CAD build for the part. Positions are in the model's coordinates, mm. A direction names the side the tool comes from. Round coordinates to 2 decimals unless told otherwise and drop trailing zeros. Loops run counter-clockwise (first coordinate to the right, second up) from the corner with the lowest first, then second, coordinate; pieces in that order, holes last. Notation, with made-up numbers: (-28.5, 79) - (-2.5, 79) arc R21 cw to (-2.5, 113) - close; hole circle Ø9 at (-7, 64). An arc over 180 degrees is marked (long way). Use one line per item in the form item = value.
from build123d import *

# Parameters (mm, degrees)
SKETCH1_W           = 53.6
SKETCH1_H           = 39.6
BOSS_EXTRUDE1_DEPTH = 2
SKETCH2_W           = 53.6
SKETCH2_H           = 39.6
SKETCH2_W_2         = 49.6
SKETCH2_H_2         = 35.6
BOSS_EXTRUDE2_DEPTH = 20
SKETCH3_W           = 70
SKETCH3_H           = 60
SKETCH3_W_2         = 49.6
SKETCH3_H_2         = 35.6
BOSS_EXTRUDE3_DEPTH = 3
CHAMFER1_SIZE       = 10
FILLET1_R           = 3


with BuildPart() as part:
    # Sketch1 → Boss-Extrude1 (new body)
    with BuildSketch(Plane(origin=(0, 0, 0), x_dir=(1, 0, 0), z_dir=(0, 1, 0))):
        Rectangle(SKETCH1_W, SKETCH1_H)
    extrude(amount=BOSS_EXTRUDE1_DEPTH)

    # Sketch2 → Boss-Extrude2 (add)
    with BuildSketch(Plane(origin=(0, 2, 0), x_dir=(1, 0, 0), z_dir=(0, 1, 0))):
        Rectangle(SKETCH2_W, SKETCH2_H)
        Rectangle(SKETCH2_W_2, SKETCH2_H_2, mode=Mode.SUBTRACT)
    extrude(amount=BOSS_EXTRUDE2_DEPTH)

    # Sketch3 → Boss-Extrude3 (add)
    with BuildSketch(Plane(origin=(0, 22, 0), x_dir=(1, 0, 0), z_dir=(0, 1, 0))):
        Rectangle(SKETCH3_W, SKETCH3_H)
        Rectangle(SKETCH3_W_2, SKETCH3_H_2, mode=Mode.SUBTRACT)
    extrude(amount=BOSS_EXTRUDE3_DEPTH)

    # Chamfer1
    chamfer1_edges = [part.edges().sort_by_distance(p)[0] for p in [
        (0, 2, -17.8),
        (0, 0, -19.8),
    ]]
    chamfer(chamfer1_edges, length=CHAMFER1_SIZE)

    # Fillet1
    fillet1_edges = [part.edges().sort_by_distance(p)[0] for p in [
        (24.8, 13.5, 17.8),
        (0, 25, 17.8),
        (-24.8, 13.5, 17.8),
        (0, 2, 17.8),
        (24.8, 18.5, -17.8),
        (-24.8, 18.5, -17.8),
        (24.8, 2, 5),
        (-24.8, 2, 5),
        (24.8, 25, 0),
        (0, 25, -17.8),
        (-24.8, 25, 0),
        (0, 25, 30),
        (0, 25, -30),
        (35, 25, 0),
        (-35, 25, 0),
        (0, 12, -17.8),
        (24.8, 7, -12.8),
        (-24.8, 7, -12.8),
        (0, 2, -7.8),
    ]]
    fillet(fillet1_edges, radius=FILLET1_R - 0.0001)  # a hair under: the kernel refuses the full size


solid = part.part
1) Flat gauge pins, fed straight in: pin 1 (11 mm diameter, centred on y = 7.5, z = -0.5, fed in from -X); pin 2 (5 mm diameter, centred on x = -9.5, y = 14, fed in from -Z); pin 3 (4 mm diameter, centred on x = 9.5, y = 15, fed in from +Z). Where does each tip first touch, or does it go through?
Report:
pin_1 = -26.8
pin_2 = -19.8
pin_3 = 19.8
2) Slice it at A-A (y = 15). Write the cut outline in (x, z), plus the area to 3 significant figures.
Report:
outline = (-26.8, -19.8) - (26.8, -19.8) - (26.8, 19.8) - (-26.8, 19.8) - close; hole (-24.8, -14.8) arc R3 ccw to (-21.8, -17.8) - (21.8, -17.8) arc R3 ccw to (24.8, -14.8) - (24.8, 14.8) arc R3 ccw to (21.8, 17.8) - (-21.8, 17.8) arc R3 ccw to (-24.8, 14.8) - close
area = 365 mm^2
3) Two-plate mould, pull along Z, no slides. Class faces 1 (the cylindrical face through (23.9, 2.86, 3.97)), 2 (the flat face through (0, 11, 19.8)), 3 (the flat face through (-0.4, 5.1, -14.9)): +Z half, -Z half, draft (parallel to the pull), parting line (faces both ways), or undercut.
Report:
face_1 = undercut
face_2 = +Z half
face_3 = -Z half
4) Slice it at D-D (y = 23). Write the cut outline in (x, z).
Report:
outline = (-34.83, -29.83) - (34.83, -29.83) - (34.83, 29.83) - (-34.83, 29.83) - close; hole (-24.97, -14.8) arc R3.17 ccw to (-21.8, -17.97) - (21.8, -17.97) arc R3.17 ccw to (24.97, -14.8) - (24.97, 14.8) arc R3.17 ccw to (21.8, 17.97) - (-21.8, 17.97) arc R3.17 ccw to (-24.97, 14.8) - close
5) Tool access for faces 4 (the flat face through (-24.8, 13, 0)), 5 (the cylindrical face through (0.49, 24.14, -29.1)), 6 (the flat face through (0, 22, -20)): list every direction of +Z, -Z, +X, -X, +Y, -Y with a clear straight run to the whole face (end or side of a thin tool).
Report:
face_4 = +Y
face_5 = -Z, +X, -X, +Y
face_6 = -Y
6) Drill centre lines: probe 1 along X at (y, z) = (9.25, 6); probe 2 along Z at (x, y) = (20, 18.5); probe 3 along Z at (x, y) = (-26, 21). Where is each one in solid material? Low to high.
Report:
probe_1 = -26.8 to -24.8, 24.8 to 26.8
probe_2 = -19.8 to -17.8, 17.8 to 19.8
probe_3 = -19.8 to 19.8
